Can you work these out from the model? Positions are in its coordinate system, mm. Face numbers are marked on the shaded views. A direction names the side the tool comes from. Coordinates: 2 decimals unless noted, no trailing zeros. Loops run counter-clockwise (first coordinate to the right, second up) from the corner with the lowest first, then second, coordinate; pieces in that order, holes last.
```python
from build123d import *

# Parameters (mm, degrees)
SKETCH_1_W               = 170
SKETCH_1_H               = 66
EXTRUDE_1_DEPTH          = 70
SKETCH_2_W               = 170
SKETCH_2_H               = 106
EXTRUDE_2_DEPTH          = 5
FILLET_1_R               = 3
SHELL_1_T                = -1.5
CUT_EXTRUDE_1_DEPTH      = 204.502456988
CUT_EXTRUDE_1_DEPTH_BACK = 5
SKETCH_3_W               = 3.5
SKETCH_3_H               = 106
SKETCH_4_R               = 11
CUT_EXTRUDE_2_DEPTH      = 5
SKETCH_5_R               = 3
CUT_EXTRUDE_3_DEPTH      = 5
FILLET_2_R               = 3


with BuildPart() as part:
    # 草图1 → 凸台-拉伸1 (new body)
    with BuildSketch(Plane.XY):
        with Locations((85, 33)):
            Rectangle(SKETCH_1_W, SKETCH_1_H)
    extrude(amount=EXTRUDE_1_DEPTH)

    # 草图2 → 凸台-拉伸2 (add)
    with BuildSketch(Plane.XY.offset(70)):
        with Locations((85, 33)):
            Rectangle(SKETCH_2_W, SKETCH_2_H)
    extrude(amount=EXTRUDE_2_DEPTH)

    # 圆角1
    fillet_1_edges = [part.edges().sort_by_distance(p)[0] for p in [
        (85, 0, 70),
        (85, 0, 0),
        (85, 66, 0),
        (85, 66, 70),
    ]]
    fillet(fillet_1_edges, radius=FILLET_1_R)

    # 抽壳1
    shell_1_openings = [part.faces().sort_by_distance(p)[0] for p in [
        (85, -20, 72.5),
        (85, 86, 72.5),
        (85, 33, 75),
    ]]
    offset(amount=SHELL_1_T, openings=shell_1_openings, kind=Kind.INTERSECTION)

    # 草图3 → 切除-拉伸1 (cut, two sides: drawn at the far end of the back side and taken through both)
    with BuildSketch(Plane.ZY.offset(-168.5).offset(-CUT_EXTRUDE_1_DEPTH_BACK)):
        with Locations((73.25, 33)):
            Rectangle(SKETCH_3_W, SKETCH_3_H)
    extrude(amount=CUT_EXTRUDE_1_DEPTH + CUT_EXTRUDE_1_DEPTH_BACK, mode=Mode.SUBTRACT)

    # 草图4 → 切除-拉伸2 (cut)
    with BuildSketch(Plane(origin=(0, 0, 0), x_dir=(-1, 0, 0), z_dir=(0, 0, -1))):
        with Locations((-135, 33)):
            Circle(SKETCH_4_R)
        with Locations((-85, 33)):
            Circle(SKETCH_4_R)
        with Locations((-35, 33)):
            Circle(SKETCH_4_R)
    extrude(amount=-CUT_EXTRUDE_2_DEPTH, mode=Mode.SUBTRACT)

    # 草图5 → 切除-拉伸3 (cut)
    with BuildSketch(Plane.XY.offset(71.5)):
        with Locations((145, -12)):
            Circle(SKETCH_5_R)
        with Locations((25, -12)):
            Circle(SKETCH_5_R)
        with Locations((25, 78)):
            Circle(SKETCH_5_R)
        with Locations((145, 78)):
            Circle(SKETCH_5_R)
    extrude(amount=-CUT_EXTRUDE_3_DEPTH, mode=Mode.SUBTRACT)

    # 圆角2
    fillet_2_edges = [part.edges().sort_by_distance(p)[0] for p in [
        (170, 86, 70.75),
        (0, 86, 70.75),
        (0, -20, 70.75),
        (170, -20, 70.75),
    ]]
    fillet(fillet_2_edges, radius=FILLET_2_R)


solid = part.part
```
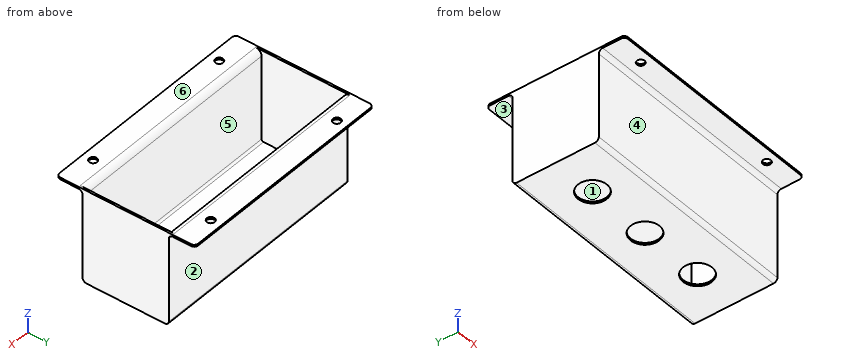
(1) If I drill on probe 1 along Y at (x, z) = (29.5, 23); probe 2 along X at (y, z) = (40, 20.5); probe 3 along Z at (x, y) = (101.5, 35.5), over which ranges is the centre line in solid material (lowest first)?
Check values:
probe 1: y = 0 to 1.5, 64.5 to 66
probe 2: x = 0 to 1.5, 168.5 to 170
probe 3: z = 0 to 1.5
(2) I'm going to push flat-ended pins straight in: pin 1 (19 mm diameter, centred on x = 119.5, z = 19.5, fed in from +Y); pin 2 (5.5 mm diameter, centred on x = 25, y = -12, fed in from -Z); pin 3 (5 mm diameter, centred on x = 89, y = 78, fed in from -Z); pin 4 (6 mm diameter, centred on x = 47.5, z = 43, fed in from -Y). Where does each tip first touch, or does it pass through?
Check values:
pin 1: stops at y = 66
pin 2: passes through
pin 3: stops at z = 70
pin 4: stops at y = 0
(3) If we mould it in two halves opening along Y, with no side actions, what happens to the marked faces 1, 2 and 3? For each: released by +Y, released by -Y, zero draft, split by the parting line, or undercut.
Check values:
face 1: undercut
face 2: released by +Y
face 3: zero draft
(4) I want a section at B-B on y = 33. Write out the boundary of the cut face in (x, z), then the cut area to 3 significant figures.
Check values:
outline: (0, 0) - (24, 0) - (24, 1.5) - (1.5, 1.5) - (1.5, 71.5) - (0, 71.5) - close; (46, 0) - (74, 0) - (74, 1.5) - (46, 1.5) - close; (96, 0) - (124, 0) - (124, 1.5) - (96, 1.5) - close; (146, 0) - (170, 0) - (170, 71.5) - (168.5, 71.5) - (168.5, 1.5) - (146, 1.5) - close
area: 366 mm2
(5) Which directions (+Z, -Z, +X, -X, +Y, -Y) give clear straight access to the entire face, cutting with the end or side of a thin tool? Please do the marked faces 4, 5 and 6.
Check values:
face 4: -Z, +X, -X, -Y
face 5: +Z
face 6: +Z, +X, -X, +Y, -Y
(6) I want a section at C-C on x = 76.5. Write out the boundary of the cut face in (y, z).
Check values:
outline: (-20, 70) - (-3, 70) arc R3 cw to (0, 67) - (0, 3) arc R3 ccw to (3, 0) - (26.02, 0) - (26.02, 1.5) - (3, 1.5) arc R1.5 cw to (1.5, 3) - (1.5, 67) arc R4.5 ccw to (-3, 71.5) - (-20, 71.5) - close; (39.98, 0) - (63, 0) arc R3 ccw to (66, 3) - (66, 67) arc R3 cw to (69, 70) - (86, 70) - (86, 71.5) - (69, 71.5) arc R4.5 ccw to (64.5, 67) - (64.5, 3) arc R1.5 cw to (63, 1.5) - (39.98, 1.5) - close
(7) I want a section at A-A on z = 58. Write out the boundary of the cut face in (x, y).
Check values:
outline: (0, 0) - (170, 0) - (170, 66) - (0, 66) - close; hole (1.5, 1.5) - (168.5, 1.5) - (168.5, 64.5) - (1.5, 64.5) - close
(8) I want a section at D-D on x = 105.5. Write out the boundary of the cut face in (y, z), then the cut area to 3 significant figures.
Check values:
outline: (-20, 70) - (-3, 70) arc R3 cw to (0, 67) - (0, 3) arc R3 ccw to (3, 0) - (63, 0) arc R3 ccw to (66, 3) - (66, 67) arc R3 cw to (69, 70) - (86, 70) - (86, 71.5) - (69, 71.5) arc R4.5 ccw to (64.5, 67) - (64.5, 3) arc R1.5 cw to (63, 1.5) - (3, 1.5) arc R1.5 cw to (1.5, 3) - (1.5, 67) arc R4.5 ccw to (-3, 71.5) - (-20, 71.5) - close
area: 361 mm2
